from build123d import *

# Parameters (mm, degrees)
F1_R          = 2
F4_DEPTH      = 2
F4_DEPTH_BACK = 2
F6_DEPTH      = 11


with BuildPart() as f2:
    # F1 (on Front) → F2 (revolve)
    with BuildSketch(Plane.XZ):
        with Locations((18, 0)):
            Circle(F1_R)
    revolve(axis=Axis((0, 0, 0), (0, 0, 1)))

    # F3 (on face) → F4 (join, two sides)
    with BuildSketch(Plane.XY) as f4_sk:
        Polygon((4, 20.003311336), (0, 20.003311336), (-4, 20.003311336), (-4, 6.003311336), (0, 6.003311336), (4, 6.003311336), align=None)
    extrude(amount=F4_DEPTH)
    extrude(f4_sk.sketch, amount=-F4_DEPTH_BACK)

    # F5 (on face) → F6 (cut)
    with BuildSketch(Plane(origin=(0, 20.003311336, 0), x_dir=(-1, 0, 0), z_dir=(0, 1, 0))):
        Polygon((-0.005, 0), (-2.005, -2), (2.005, -2), (0.005, 0), (2.005, 2), (-2.005, 2), align=None)
    extrude(amount=-F6_DEPTH, mode=Mode.SUBTRACT)


solid = f2.part
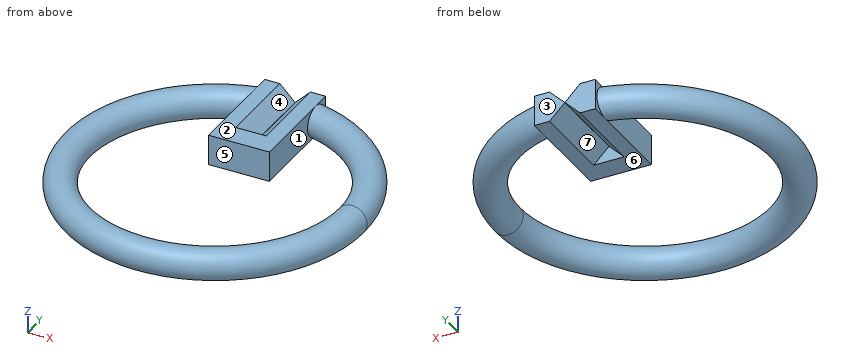
Could you check a few things on this model? Use its own coordinates, in mm. Face numbers are marked on the shaded views. A direction names the side the tool comes from. Coordinates: 2 decimals unless noted, no trailing zeros. Order: outer loops, then holes, each group sorted by start corner. A loop starts at its lowest first (then second) coordinate and runs counter-clockwise, first axis right, second up.
Q1. Which directions (+Z, -Z, +X, -X, +Y, -Y) give clear straight access to the entire face, cutting with the end or side of a thin tool? Please do the marked faces 4, 5, 6 and 7.
Q2. Suppose I cut it at A-A on z = -1.15. Please give me the cut outline in (x, y) (3 decimals), and give its area (3 significant figures).
Q3. Please list where these lines run through material, in increasing order: L1, parallel to X at y = 12.5, z = 1.4 (3 decimals); L2, parallel to Z at x = 8, y = -16; L3, parallel to Y at x = 4.5, z = 1.75.
Q4. Will these pins go through, and if not, where does the flat tip stop? pin 1 (2 mm diameter, centred on y = 12, z = -0.5, fed in from +X); pin 2 (1.5 mm diameter, centred on y = -4.5, z = -1, fed in from -X); pin 3 (2 mm diameter, centred on y = 18.5, z = 1, fed in from -X).
Q5. Thinking about a two-plate mould opening in Y: for the marked faces 1, 2 and 3, which applies, released by +Y, released by -Y, zero draft, split by the parting line, or undercut?
Q6. Suppose I cut it at C-C on z = 1.2. Please give me the cut outline in (x, y) (1 decimal), and give its area (3 significant figures).
Q7. Suppose I cut it at B-B on y = 10.5. Give the number of separate pieces and of enclosed holes in the cut face, and give its area (3 significant figures).
Answer:
1. face 4: +Z, +Y
1. face 5: +Z, -Z
1. face 6: -Z, +X, -X, +Y, -Y
1. face 7: -Z, +Y
2. outline: (-4, 19.225) arc R19.636 ccw (long way) to (4, 19.225) - (4, 20.003) - (1.155, 20.003) - (1.155, 9.003) - (-1.155, 9.003) - (-1.155, 20.003) - (-4, 20.003) - close; hole (-4, 6.003) - (-4, 15.867) arc R16.364 ccw (long way) to (4, 15.867) - (4, 6.003) - close
2. area: 430 mm2
3. L1: x = -14.873 to -10.88, -4 to -1.405, 1.405 to 4, 10.88 to 14.873
3. L2: z = -2 to 2
3. L3: y = -18.43 to -16.43, 16.43 to 18.43
4. pin 1: stops at x = 16.66
4. pin 2: stops at x = -19.55
4. pin 3: stops at x = -9.34
5. face 1: undercut
5. face 2: zero draft
5. face 3: released by +Y
6. outline: (-4, 19.2) arc R19.6 ccw (long way) to (4, 19.2) - (4, 20) - (1.2, 20) - (1.2, 9) - (-1.2, 9) - (-1.2, 20) - (-4, 20) - close; hole (-4, 6) - (-4, 15.9) arc R16.4 ccw (long way) to (4, 15.9) - (4, 6) - close
6. area: 422 mm2
7. separate pieces: 4
7. enclosed holes: 0
7. area: 55.0 mm2
